Check sheet for the modelled part. Datum: model origin and axes. Units: mm. A direction names the side the tool comes from. Give positions to 0.01 mm unless a question says otherwise; leave off trailing zeros. Order: outer loops, then holes, each group sorted by start corner. A loop starts at its lowest first (then second) coordinate and runs counter-clockwise, first axis right, second up. Notation, with made-up numbers: (67.25, 1) -> (119.25, 1) arc R15 cw to (119.25, 22) -> close; hole circle Ø4 at (0, 3.25). An arc over 180 degrees is marked (long way). Answer in a Markdown table with one row per item. Add a question column.
(1) Release check for a two-part mould opening along X. For faces 3 (the face through (-2, 2, -10)), 4 (the face through (66.89, -58.78, -7.46)), 5 (the face through (49.73, -67.91, -4.76)), 6 (the face through (-124.88, 5.5, -8.99)) record: released by +X, released by -X, zero draft, split by the parting line, or undercut.
(2) Thickness scan on L1, parallel to Z at x = 54, y = -19.5; L2, parallel to X at y = 105.5, z = 120; L3, parallel to Y at x = 30.5, z = 264.5. Record the ranges inside material, lowest first. Write a range as [from, to].
(3) Cross-section at A-A (z = 184). Record the cut outline in (x, y), then the cut area to 3 significant figures.
(4) Go/stop test with flat-tipped pins: pin 1 (6 mm diameter, centred on x = -36.5, z = 277, fed in from -Y); pin 2 (4 mm diameter, centred on x = 23.5, z = 75.5, fed in from -Y); pin 3 (6 mm diameter, centred on x = -37, z = 194.5, fed in from -Y). Record where each tip stops, or that it passes through.
(5) Set-up check for faces 1 (the face through (-2, 2, 0)), 2 (the face through (35, 90, 322)): record each of +Z, -Z, +X, -X, +Y, -Y from which the full face is reachable in a straight line by a thin tool's end or side.
(6) Cross-section at B-B (y = 5.5). State how many separate pieces and enclosed holes the cut face has, then the cut area to 3 significant figures.
```python
from build123d import *

# Parameters (mm, degrees)
F1_R     = 125
F1_R_2   = 15
F2_DEPTH = 10
F3_R     = 8
F4_SIZE  = 5
F5_R     = 17.149264
F5_R_2   = 18.207102
F5_R_3   = 18.26978
F5_R_4   = 17.319041
F6_DEPTH = 322


with BuildPart() as f2:
    # F1 (on face) → F2 (new body)
    with BuildSketch(Plane.XY):
        Circle(F1_R)
        with Locations((-53.033009, -53.033009)):
            Circle(F1_R_2, mode=Mode.SUBTRACT)
        with Locations((0, -75)):
            Circle(F1_R_2, mode=Mode.SUBTRACT)
        with Locations((53.033009, -53.033009)):
            Circle(F1_R_2, mode=Mode.SUBTRACT)
        with Locations((-75, 0)):
            Circle(F1_R_2, mode=Mode.SUBTRACT)
        with Locations((-53.033009, 53.033009)):
            Circle(F1_R_2, mode=Mode.SUBTRACT)
        with Locations((53.033009, 53.033009)):
            Circle(F1_R_2, mode=Mode.SUBTRACT)
        with Locations((75, 0)):
            Circle(F1_R_2, mode=Mode.SUBTRACT)
        with Locations((0, 75)):
            Circle(F1_R_2, mode=Mode.SUBTRACT)
    extrude(amount=-F2_DEPTH)

    # F3
    f3_edges = [f2.edges().sort_by_distance(p)[0] for p in [
        (-125, 0, 0),
    ]]
    fillet(f3_edges, radius=F3_R)

    # F4
    f4_edges = [f2.edges().sort_by_distance(p)[0] for p in [
        (-68.033009, 53.033009, 0),
        (-15, 75, 0),
        (-90, 0, 0),
        (38.033009, 53.033009, 0),
        (-68.033009, -53.033009, 0),
        (-15, -75, 0),
        (38.033009, -53.033009, 0),
        (60, 0, 0),
    ]]
    chamfer(f4_edges, length=F4_SIZE)

    # F5 (on face) → F6 (join)
    with BuildSketch(Plane.XY):
        with Locations((-40.163934, -90.607919)):
            Circle(F5_R)
        with Locations((36.81694, -90.607919)):
            Circle(F5_R_2)
        with Locations((35.382513, 90.129778)):
            Circle(F5_R_3)
        with Locations((-40.163934, 89.651637)):
            Circle(F5_R_4)
    extrude(amount=F6_DEPTH)


solid = f2.part
```
Answer below:
| question | item | result |
|---|---|---|
| 1 | face 3 | zero draft |
| 1 | face 4 | undercut |
| 1 | face 5 | undercut |
| 1 | face 6 | split by the parting line |
| 2 | L1 | z = [-10, 0] |
| 2 | L2 | x = [-47.15, -33.18], [25.51, 45.26] |
| 2 | L3 | y = [-107.68, -73.53], [72.52, 107.74] |
| 3 | outline | circle Ø34.64 at (-40.16, 89.65); circle Ø34.3 at (-40.16, -90.61); circle Ø36.54 at (35.38, 90.13); circle Ø36.41 at (36.82, -90.61) |
| 3 | area | 3,960 mm² |
| 4 | pin 1 | stops at y = -107.74 |
| 4 | pin 2 | stops at y = -104.87 |
| 4 | pin 3 | stops at y = -107.76 |
| 5 | face 1 | +Z |
| 5 | face 2 | +Z, +X, -X, +Y, -Y |
| 6 | separate pieces | 3 |
| 6 | enclosed holes | 0 |
| 6 | area | 1,860 mm² |
